The figure shows three views and two pictorial views of one solid part (mm, origin at its lowest corner). Answer the questions. A direction names the side the tool comes from. Coordinates: 2 decimals unless noted, no trailing zeros. Order: outer loops, then holes, each group sorted by start corner. A loop starts at its lowest first (then second) coordinate and runs counter-clockwise, first axis right, second up.
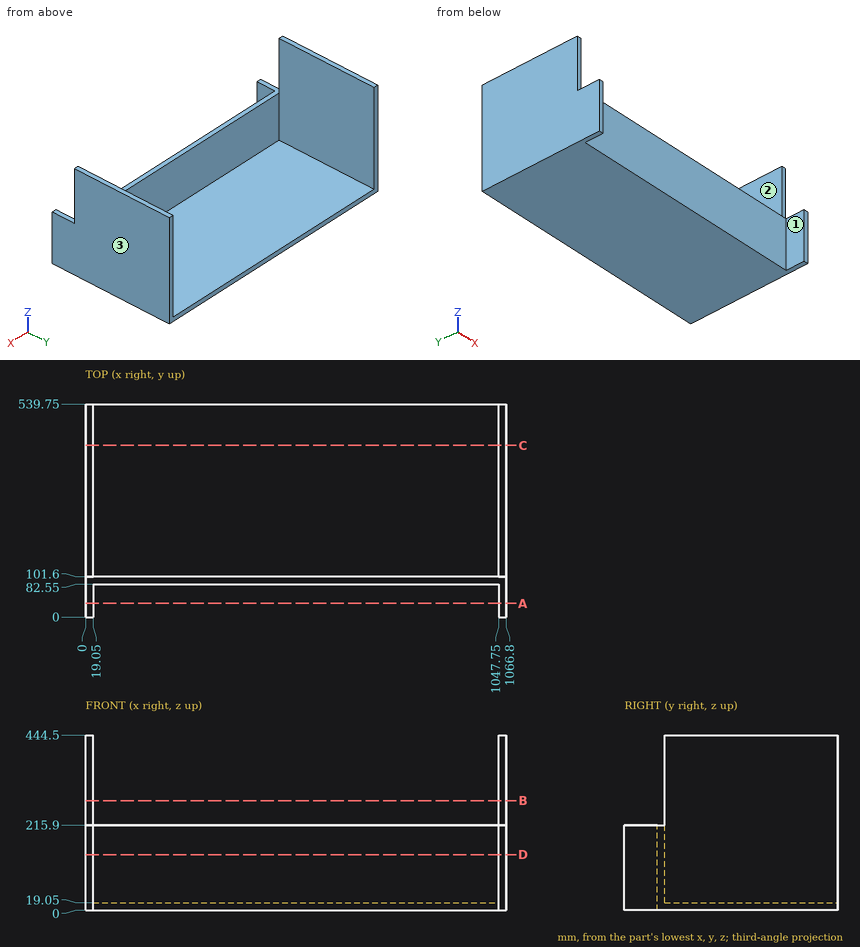
1) A cutting plane is placed at B-B, the plane z = 278.5. Write down the section's boundary in (x, y).
2) A cutting plane is placed at C-C, the plane y = 435. Write down the section's boundary in (x, z).
3) A cutting plane is placed at D-D, the plane z = 141.5. Write down the section's boundary in (x, y).
4) For the marked faces 1, 2 and 3, determine the directions among +Z, -Z, +X, -X, +Y, -Y from which every point of the face is accessible in a straight line to the end or side of a thin tool.
5) A cutting plane is placed at A-A, the plane y = 34.5. Write down the section's boundary in (x, z), plus the area to 3 significant figures.
6) Each of these flat-tipped pins is pushed along its axis until it touches: P1, Ø1.5, axis at x = 352.5, y = 398, coming from the +Z side; P2, Ø21, axis at x = 1057, z = 285.5, coming from the -Y side; P3, Ø1, axis at x = 647, z = 202, coming from the -Y side. Where does it stop, or does it pass through?
7) Straight lines are drawn through the part: probe 1 along X at (y, z) = (316, 278); probe 2 along Z at (x, y) = (871, 105.5); probe 3 along Y at (x, z) = (807.5, 67). For each, find the intervals that lie inside material, in ascending order.
Working result:
1. outline: (0, 101.6) - (19.05, 101.6) - (19.05, 539.75) - (0, 539.75) - close; (1047.75, 101.6) - (1066.8, 101.6) - (1066.8, 539.75) - (1047.75, 539.75) - close
2. outline: (0, 0) - (1066.8, 0) - (1066.8, 444.5) - (1047.75, 444.5) - (1047.75, 19.05) - (19.05, 19.05) - (19.05, 444.5) - (0, 444.5) - close
3. outline: (0, 0) - (19.05, 0) - (19.05, 82.55) - (1047.75, 82.55) - (1047.75, 0) - (1066.8, 0) - (1066.8, 539.75) - (1047.75, 539.75) - (1047.75, 101.6) - (19.05, 101.6) - (19.05, 539.75) - (0, 539.75) - close
4. face 1: +Z, -Z, -Y
4. face 2: +Z, +Y
4. face 3: +Z, -Z, +X, +Y, -Y
5. outline: (0, 0) - (19.05, 0) - (19.05, 215.9) - (0, 215.9) - close; (1047.75, 0) - (1066.8, 0) - (1066.8, 215.9) - (1047.75, 215.9) - close
5. area: 8,230 mm2
6. P1: stops at z = 19.05
6. P2: stops at y = 101.6
6. P3: stops at y = 82.55
7. probe 1: x = 0 to 19.05, 1047.75 to 1066.8
7. probe 2: z = 0 to 19.05
7. probe 3: y = 82.55 to 101.6
